Read the model definition and answer for the solid it produces. Units are mm, in the model's axes. A direction names the side the tool comes from. Give positions to 0.01 mm unless a question says otherwise; leave off trailing zeros. Order: outer loops, then holes, each group sorted by start corner. A loop starts at its lowest first (then second) coordinate and runs counter-clockwise, first axis right, second up. Notation, with made-up numbers: M -30,43.5 L 14,43.5 A26 ccw 14,74.5 Z; hole C 89.5,53.5 d9. An arc over 180 degrees is marked long. One line per item, written item: value.
from build123d import *

# Parameters (mm, degrees)
SKETCH1_W           = 27
SKETCH1_H           = 50
BOSS_EXTRUDE1_DEPTH = 10
SKETCH2_R           = 3.5
CUT_EXTRUDE1_DEPTH  = 10
SKETCH3_R           = 5.5
CUT_EXTRUDE2_DEPTH  = 7
BOSS_EXTRUDE2_DEPTH = 4


with BuildPart() as part:
    # Sketch1 → Boss-Extrude1 (new body)
    with BuildSketch(Plane(origin=(0, 0, 0), x_dir=(0, 0, -1), z_dir=(1, 0, 0))):
        with Locations((0, -15)):
            Rectangle(SKETCH1_W, SKETCH1_H)
    extrude(amount=BOSS_EXTRUDE1_DEPTH)

    # Sketch2 → Cut-Extrude1 (cut)
    with BuildSketch(Plane(origin=(10, 0, 0), x_dir=(0, 0, -1), z_dir=(1, 0, 0))):
        Circle(SKETCH2_R)
    extrude(amount=-CUT_EXTRUDE1_DEPTH, mode=Mode.SUBTRACT)

    # Sketch3 → Cut-Extrude2 (cut)
    with BuildSketch(Plane(origin=(10, 0, 0), x_dir=(0, 0, -1), z_dir=(1, 0, 0))):
        Circle(SKETCH3_R)
    extrude(amount=-CUT_EXTRUDE2_DEPTH, mode=Mode.SUBTRACT)

    # Sketch4 → Boss-Extrude2 (add)
    with BuildSketch(Plane.XY.offset(13.5)):
        with BuildLine():
            Line((10, 0), (19, 0))
            Line((19, 0), (19, 0.8))
            ThreePointArc((19, 0.8), (19.292893219, 1.507106781), (20, 1.8))
            Line((20, 1.8), (20.6, 1.8))
            ThreePointArc((20.6, 1.8), (21.307106781, 1.507106781), (21.6, 0.8))
            Line((21.6, 0.8), (21.6, -3.5))
            ThreePointArc((21.6, -3.5), (21.307106781, -4.207106781), (20.6, -4.5))
            Line((20.6, -4.5), (10, -4.5))
            Line((10, -4.5), (10, 0))
        make_face()
        with BuildLine():
            Line((10, -30.9), (19, -30.9))
            Line((19, -30.9), (19, -30.1))
            ThreePointArc((19, -30.1), (19.292893219, -29.392893219), (20, -29.1))
            Line((20, -29.1), (20.6, -29.1))
            ThreePointArc((20.6, -29.1), (21.307106781, -29.392893219), (21.6, -30.1))
            Line((21.6, -30.1), (21.6, -34.4))
            ThreePointArc((21.6, -34.4), (21.307106781, -35.107106781), (20.6, -35.4))
            Line((20.6, -35.4), (10, -35.4))
            Line((10, -35.4), (10, -30.9))
        make_face()
    boss_extrude2 = extrude(amount=-BOSS_EXTRUDE2_DEPTH)

    # Mirror1: Boss-Extrude2 across plane
    add(boss_extrude2.mirror(Plane.XY))


solid = part.part
1) Which of the six approach directions +Z, -Z, +X, -X, +Y, -Y give full straight-line access (tool end or side, diameter ignored) to faces 1 (the face through (16, -33, -9.5)), 2 (the face through (14, 0, -12)), 3 (the face through (15, -35.4, -12)), 4 (the face through (6.55, -5.37, 1.19)), 5 (the face through (15, -4.5, -12))?
Reported:
face 1: +X, +Y, -Y
face 2: +Z, -Z, +Y
face 3: +Z, -Z, +X, -Y
face 4: +X
face 5: +Z, -Z, +X
2) Find section B-B, the plane x = 12.5. Write down the section's boundary in (y, z), plus the area to 3 significant figures.
Reported:
outline: M -35.4,-13.5 L -30.9,-13.5 L -30.9,-9.5 L -35.4,-9.5 Z; M -35.4,9.5 L -30.9,9.5 L -30.9,13.5 L -35.4,13.5 Z; M -4.5,-13.5 L 0,-13.5 L 0,-9.5 L -4.5,-9.5 Z; M -4.5,9.5 L 0,9.5 L 0,13.5 L -4.5,13.5 Z
area: 72.0 mm^2
3) Find section A-A, the plane z = 0. Write down the section's boundary in (x, y), plus the area to 3 significant figures.
Reported:
outline: M 0,-40 L 10,-40 L 10,-5.5 L 3,-5.5 L 3,-3.5 L 0,-3.5 Z; M 0,3.5 L 3,3.5 L 3,5.5 L 10,5.5 L 10,10 L 0,10 Z
area: 402 mm^2
4) Each of these flat-tipped pins is pushed along its axis until it touches: pin 1 Ø1 at (y, z) = (-29, -3) entering from +X; pin 2 Ø1 at (x, z) = (16.5, -10.5) entering from +Y; pin 3 Ø2 at (x, z) = (14.5, -11.5) entering from -Y. Where does it stop, or does it pass through?
Reported:
pin 1: stops at x = 10
pin 2: stops at y = 0
pin 3: stops at y = -35.4
5) Find section D-D, the plane x = 5.25. Write down the section's boundary in (y, z).
Reported:
outline: M -40,-13.5 L 10,-13.5 L 10,13.5 L -40,13.5 Z; hole C 0,0 d11
6) Determine the mould class of faces 6 (the face through (14, -30.9, 12)), 7 (the face through (21.6, -32, 12)), 8 (the face through (16, -2, 9.5)) for opening direction X: +X half, -X half, draft (parallel to the pull), parting line (faces both ways), or undercut.
Reported:
face 6: undercut
face 7: +X half
face 8: draft
7) Find section C-C, the plane z = -4.5. Write down the section's boundary in (x, y), plus the area to 3 significant figures.
Reported:
outline: M 0,-40 L 10,-40 L 10,-3.16 L 3,-3.16 L 3,3.16 L 10,3.16 L 10,10 L 0,10 Z
area: 456 mm^2
8) Consider probe 1 along Y at (x, z) = (4.5, 0); probe 2 along Z at (x, y) = (12.75, -33); probe 3 along Y at (x, z) = (2.1, 0). Determine where each line is inside the solid, lowest interval first.
Reported:
probe 1: y = -40 to -5.5, 5.5 to 10
probe 2: z = -13.5 to -9.5, 9.5 to 13.5
probe 3: y = -40 to -3.5, 3.5 to 10
